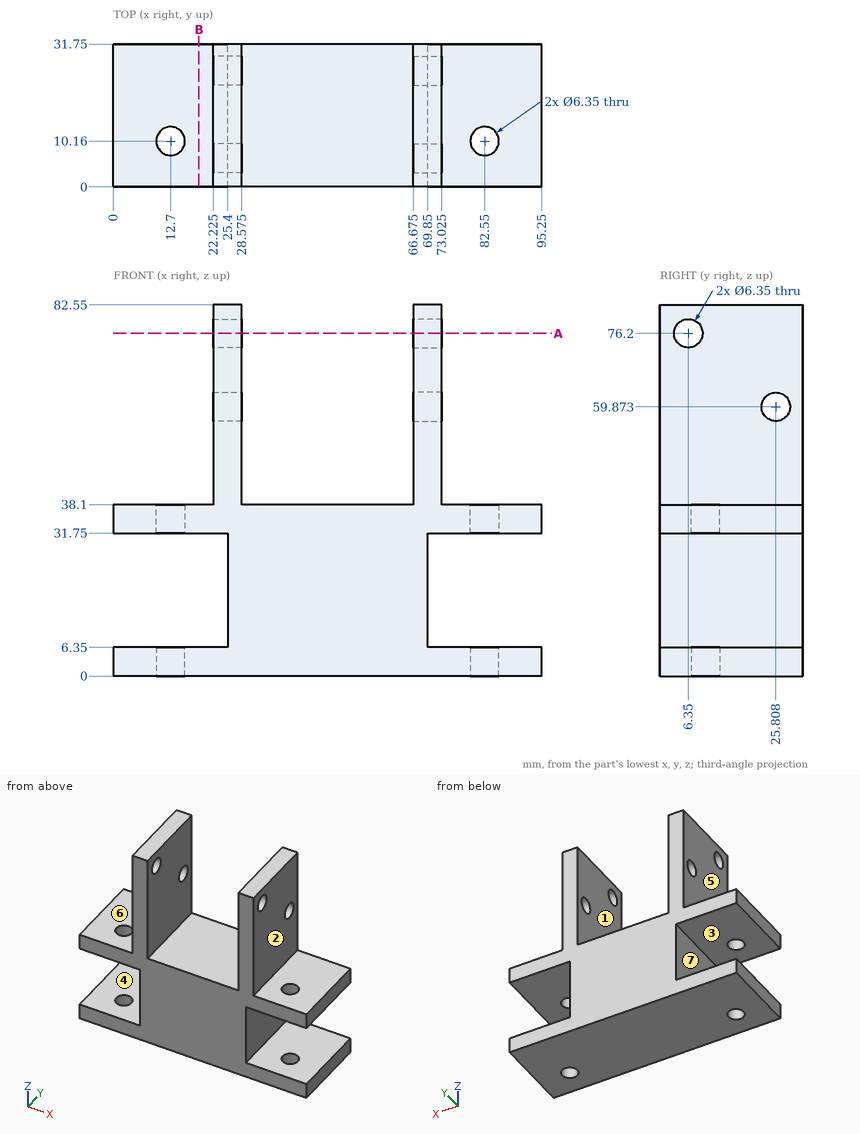
Geometry check sheet. Reference: drawing and pictorial views, mm from the part's lowest x, y, z. A direction names the side the tool comes from. Coordinates: 2 decimals unless noted, no trailing zeros. Loops run counter-clockwise (first coordinate to the right, second up) from the corner with the lowest first, then second, coordinate; pieces in that order, holes last. Notation, with made-up numbers: (17, 69.5) -> (75, 69.5) arc R12 cw to (75, 82.5) -> close; hole circle Ø1 at (12.25, 53). An arc over 180 degrees is marked (long way). Write item = value, one per line. Start each with the question number.
1. Tool access check on the marked faces 1, 2 and 3. Record the directions out of +Z, -Z, +X, -X, +Y, -Y that give a thin tool (end or side, any length) a straight path to the whole face; none if there is none.
2. Draft check along Z on the marked faces 4, 5, 6 and 7. Enter one of: released by +Z, released by -Z, zero draft, split by the parting line, or undercut.
3. Section check B-B on x = 19. Record the cut outline in (y, z).
4. Depth check by flat-ended pin: P1, Ø4, axis at y = 6.35, z = 76.2, coming from the -X side; P2, Ø18, axis at x = 89.5, y = 21.5, coming from the +Z side; P3, Ø16, axis at y = 9.5, z = 69.5, coming from the +X side (3 decimals); P4, Ø9.5, axis at y = 12.5, z = 71, coming from the -X side (3 decimals). Enter the tip coordinate at first touch or a pass-through.
5. Section check A-A on z = 76.2. Give the number of separate pieces and of enclosed holes in the cut face.
6. Material ranges on line 1 (Z direction, x = 6.5, y = 8); line 2 (Z direction, x = 71, y = 19.5); line 3 (X direction, y = 5, z = 55.5) (1 decimal), recorded low to high.
Responses:
q1.face_1 = +Z, +Y, -Y
q1.face_2 = +Z, +X, +Y, -Y
q1.face_3 = -X, +Y, -Y
q2.face_4 = undercut
q2.face_5 = zero draft
q2.face_6 = released by +Z
q2.face_7 = undercut
q3.outline = (0, 0) -> (31.75, 0) -> (31.75, 6.35) -> (0, 6.35) -> close; (0, 31.75) -> (31.75, 31.75) -> (31.75, 38.1) -> (0, 38.1) -> close
q4.P1 = through
q4.P2 = 38.1
q4.P3 = 73.025
q4.P4 = 22.225
q5.separate_pieces = 4
q5.enclosed_holes = 0
q6.line_1 = 0 to 6.35, 31.75 to 38.1
q6.line_2 = 0 to 6.35, 31.75 to 82.55
q6.line_3 = 22.2 to 28.6, 66.7 to 73
